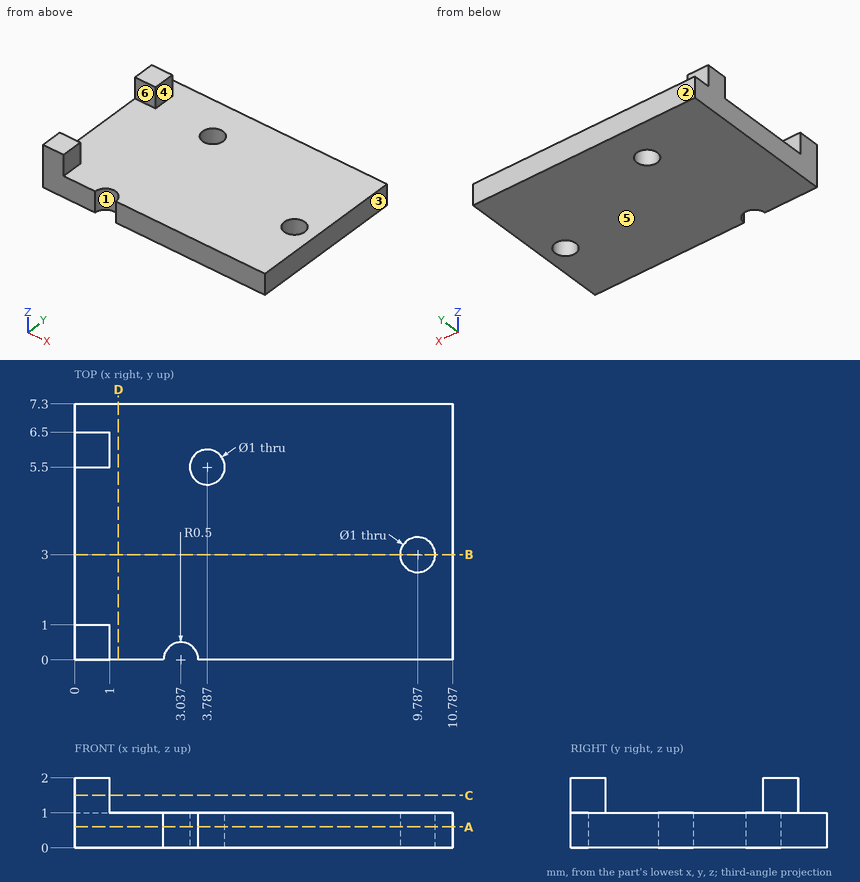
Geometry check sheet. Reference: drawing and pictorial views, mm from the part's lowest x, y, z. A direction names the side the tool comes from. Give positions to 0.01 mm unless a question says otherwise; leave off trailing zeros. Order: outer loops, then holes, each group sorted by start corner. A loop starts at its lowest first (then second) coordinate and runs counter-clockwise, first axis right, second up. Notation, with made-up numbers: M 1.5,79.5 L 46.5,79.5 A18 cw 46.5,108.5 Z; hole C 14,51 d4. An arc over 180 degrees is marked long. Return JSON: item names as keys, results as strings. Group by question number.
1) Access from +Z, -Z, +X, -X, +Y, -Y to the whole of each face (thin tool, end or side, straight path). Record for the marked faces 4, 5 and 6.
2) Section check B-B on y = 3. Record the cut outline in (x, z).
3) Section check A-A on z = 0.6. Record the cut outline in (x, y).
4) Go/stop test with flat-tipped pins: pin 1 Ø2 at (x, y) = (8.5, 5) entering from -Z; pin 2 Ø0.5 at (x, z) = (0.5, 1.5) entering from +Y; pin 3 Ø2 at (x, y) = (2.5, 1.5) entering from +Z. Record where each tip stops, or that it passes through.
5) Mould release check, pull along X, two halves, no side actions. Record for the marked faces 1, 2 and 3: pulls with the +X half, pulls with the -X half, needs draft (parallel to the pull), parting line crosses it, or undercut.
6) Section check C-C on z = 1.5. Record the cut outline in (x, y).
7) Scan lines: line 1 (Y direction, x = 9.75, z = 0.2); line 2 (Z direction, x = 6.5, y = 4). Record each from-to range of solid material in increasing order.
8) Section check D-D on x = 1.25. Record the cut outline in (y, z).
Answer block:
{
 "1": {"face 4": "+Z, +X, +Y, -Y", "face 5": "-Z, +X, -X, +Y, -Y", "face 6": "+Z, +X, -X"},
 "2": {"outline": "M 0,0 L 9.29,0 L 9.29,1 L 0,1 Z; M 10.29,0 L 10.79,0 L 10.79,1 L 10.29,1 Z"},
 "3": {"outline": "M 0,0 L 2.54,0 A0.5 cw 3.54,0 L 10.79,0 L 10.79,7.3 L 0,7.3 Z; hole C 3.79,5.5 d1; hole C 9.79,3 d1"},
 "4": {"pin 1": "stops at z = 0", "pin 2": "stops at y = 6.5", "pin 3": "stops at z = 1"},
 "5": {"face 1": "undercut", "face 2": "needs draft", "face 3": "pulls with the +X half"},
 "6": {"outline": "M 0,0 L 1,0 L 1,1 L 0,1 Z; M 0,5.5 L 1,5.5 L 1,6.5 L 0,6.5 Z"},
 "7": {"line 1": "y = 0 to 2.5, 3.5 to 7.3", "line 2": "z = 0 to 1"},
 "8": {"outline": "M 0,0 L 7.3,0 L 7.3,1 L 0,1 Z"}
}
